CAD build for the part. Positions are in the model's coordinates, mm. Give positions to 0.01 mm unless a question says otherwise; leave off trailing zeros. Order: outer loops, then holes, each group sorted by start corner. A loop starts at its lowest first (then second) coordinate and runs counter-clockwise, first axis right, second up.
from build123d import *

# Parameters (mm, degrees)
BOSS_EXTRUDE1_DEPTH = 6.6


with BuildPart() as part:
    # Model → Boss-Extrude1 (new body)
    with BuildSketch(Plane.XY):
        with BuildLine():
            Line((-2.7, 21.1), (0, 21.1))
            Line((0, 21.1), (0, 0))
            Line((0, 0), (-76.35, 26.1117))
            Line((-76.35, 26.1117), (-100, 49.2))
            Line((-100, 49.2), (-100, 380.9))
            Line((-100, 380.9), (-97.5, 383.4))
            Line((-97.5, 383.4), (-80, 383.4))
            Line((-80, 383.4), (-61.92031318, 366.450293606))
            Line((-61.92031318, 366.450293606), (-69.443665597, 358.42538436))
            Line((-69.443665597, 358.42538436), (-70.599982066, 359.50943105))
            ThreePointArc((-70.599982066, 359.50943105), (-70.958073277, 359.644402505), (-71.306721232, 359.486633012))
            Line((-71.306721232, 359.486633012), (-74.042485748, 356.568484196))
            ThreePointArc((-74.042485748, 356.568484196), (-74.177457203, 356.210392984), (-74.01968771, 355.861745029))
            Line((-74.01968771, 355.861745029), (-72.863371242, 354.77769834))
            Line((-72.863371242, 354.77769834), (-75.941106322, 351.494780921))
            ThreePointArc((-75.941106322, 351.494780921), (-76.076077777, 351.13668971), (-75.918308284, 350.788041755))
            Line((-75.918308284, 350.788041755), (-74.057988413, 349.043991876))
            ThreePointArc((-74.057988413, 349.043991876), (-73.699897202, 348.909020421), (-73.351249247, 349.066789913))
            Line((-73.351249247, 349.066789913), (-70.273514167, 352.349707332))
            Line((-70.273514167, 352.349707332), (-69.117197698, 351.265660643))
            ThreePointArc((-69.117197698, 351.265660643), (-68.759106487, 351.130689188), (-68.410458532, 351.288458681))
            Line((-68.410458532, 351.288458681), (-65.674694016, 354.206607497))
            ThreePointArc((-65.674694016, 354.206607497), (-65.539722561, 354.564698709), (-65.697492054, 354.913346664))
            Line((-65.697492054, 354.913346664), (-66.853808523, 355.997393353))
            Line((-66.853808523, 355.997393353), (-59.330456105, 364.022302598))
            Line((-59.330456105, 364.022302598), (-45.469249226, 351.02742115))
            Line((-45.469249226, 351.02742115), (-42.733484711, 353.945569966))
            ThreePointArc((-42.733484711, 353.945569966), (-40.990244935, 354.73441743), (-39.199788878, 354.059560154))
            Line((-39.199788878, 354.059560154), (-31.904416837, 347.220148866))
            ThreePointArc((-31.904416837, 347.220148866), (-31.115569373, 345.47690909), (-31.790426649, 343.686453033))
            Line((-31.790426649, 343.686453033), (-34.526191164, 340.768304216))
            Line((-34.526191164, 340.768304216), (-20.664984286, 327.773422768))
            Line((-20.664984286, 327.773422768), (-28.188336703, 319.748513522))
            Line((-28.188336703, 319.748513522), (-29.344653172, 320.832560211))
            ThreePointArc((-29.344653172, 320.832560211), (-29.702744383, 320.967531667), (-30.051392338, 320.809762174))
            Line((-30.051392338, 320.809762174), (-32.787156854, 317.891613357))
            ThreePointArc((-32.787156854, 317.891613357), (-32.922128309, 317.533522146), (-32.764358816, 317.184874191))
            Line((-32.764358816, 317.184874191), (-31.608042348, 316.100827502))
            Line((-31.608042348, 316.100827502), (-34.685777428, 312.817910083))
            ThreePointArc((-34.685777428, 312.817910083), (-34.820748883, 312.459818871), (-34.66297939, 312.111170916))
            Line((-34.66297939, 312.111170916), (-32.802659519, 310.367121038))
            ThreePointArc((-32.802659519, 310.367121038), (-32.444568308, 310.232149583), (-32.095920353, 310.389919075))
            Line((-32.095920353, 310.389919075), (-29.018185273, 313.672836494))
            Line((-29.018185273, 313.672836494), (-27.861868804, 312.588789805))
            ThreePointArc((-27.861868804, 312.588789805), (-27.503777593, 312.45381835), (-27.155129638, 312.611587842))
            Line((-27.155129638, 312.611587842), (-24.419365122, 315.529736659))
            ThreePointArc((-24.419365122, 315.529736659), (-24.284393667, 315.88782787), (-24.44216316, 316.236475825))
            Line((-24.44216316, 316.236475825), (-25.598479629, 317.320522515))
            Line((-25.598479629, 317.320522515), (-18.075127211, 325.34543176))
            Line((-18.075127211, 325.34543176), (0, 308.4))
            Line((0, 308.4), (0, 295.7))
            Line((0, 295.7), (-2.7, 295.7))
            Line((-2.7, 295.7), (-2.7, 280.7))
            Line((-2.7, 280.7), (0, 280.7))
            Line((0, 280.7), (0, 270.3))
            Line((0, 270.3), (-11, 270.3))
            Line((-11, 270.3), (-11, 271.885))
            ThreePointArc((-11, 271.885), (-11.146446609, 272.238553391), (-11.5, 272.385))
            Line((-11.5, 272.385), (-15.5, 272.385))
            ThreePointArc((-15.5, 272.385), (-15.853553391, 272.238553391), (-16, 271.885))
            Line((-16, 271.885), (-16, 270.3))
            Line((-16, 270.3), (-20.5, 270.3))
            ThreePointArc((-20.5, 270.3), (-20.853553391, 270.153553391), (-21, 269.8))
            Line((-21, 269.8), (-21, 267.25))
            ThreePointArc((-21, 267.25), (-20.853553391, 266.896446609), (-20.5, 266.75))
            Line((-20.5, 266.75), (-16, 266.75))
            Line((-16, 266.75), (-16, 265.165))
            ThreePointArc((-16, 265.165), (-15.853553391, 264.811446609), (-15.5, 264.665))
            Line((-15.5, 264.665), (-11.5, 264.665))
            ThreePointArc((-11.5, 264.665), (-11.146446609, 264.811446609), (-11, 265.165))
            Line((-11, 265.165), (-11, 266.75))
            Line((-11, 266.75), (0, 266.75))
            Line((0, 266.75), (0, 232.2))
            Line((0, 232.2), (4, 232.2))
            ThreePointArc((4, 232.2), (5.767766953, 231.467766953), (6.5, 229.7))
            Line((6.5, 229.7), (6.5, 219.7))
            ThreePointArc((6.5, 219.7), (5.767766953, 217.932233047), (4, 217.2))
            Line((4, 217.2), (0, 217.2))
            Line((0, 217.2), (0, 209.166666667))
            Line((0, 209.166666667), (-2.7, 209.166666667))
            Line((-2.7, 209.166666667), (-2.7, 194.166666667))
            Line((-2.7, 194.166666667), (0, 194.166666667))
            Line((0, 194.166666667), (0, 155.975))
            Line((0, 155.975), (-11, 155.975))
            Line((-11, 155.975), (-11, 157.56))
            ThreePointArc((-11, 157.56), (-11.146446609, 157.913553391), (-11.5, 158.06))
            Line((-11.5, 158.06), (-15.5, 158.06))
            ThreePointArc((-15.5, 158.06), (-15.853553391, 157.913553391), (-16, 157.56))
            Line((-16, 157.56), (-16, 155.975))
            Line((-16, 155.975), (-20.5, 155.975))
            ThreePointArc((-20.5, 155.975), (-20.853553391, 155.828553391), (-21, 155.475))
            Line((-21, 155.475), (-21, 152.925))
            ThreePointArc((-21, 152.925), (-20.853553391, 152.571446609), (-20.5, 152.425))
            Line((-20.5, 152.425), (-16, 152.425))
            Line((-16, 152.425), (-16, 150.84))
            ThreePointArc((-16, 150.84), (-15.853553391, 150.486446609), (-15.5, 150.34))
            Line((-15.5, 150.34), (-11.5, 150.34))
            ThreePointArc((-11.5, 150.34), (-11.146446609, 150.486446609), (-11, 150.84))
            Line((-11, 150.84), (-11, 152.425))
            Line((-11, 152.425), (0, 152.425))
            Line((0, 152.425), (0, 122.633333333))
            Line((0, 122.633333333), (-2.7, 122.633333333))
            Line((-2.7, 122.633333333), (-2.7, 107.633333333))
            Line((-2.7, 107.633333333), (0, 107.633333333))
            Line((0, 107.633333333), (0, 91.2))
            Line((0, 91.2), (4, 91.2))
            ThreePointArc((4, 91.2), (5.767766953, 90.467766953), (6.5, 88.7))
            Line((6.5, 88.7), (6.5, 78.7))
            ThreePointArc((6.5, 78.7), (5.767766953, 76.932233047), (4, 76.2))
            Line((4, 76.2), (0, 76.2))
            Line((0, 76.2), (0, 54.35))
            Line((0, 54.35), (-11, 54.35))
            Line((-11, 54.35), (-11, 55.935))
            ThreePointArc((-11, 55.935), (-11.146446609, 56.288553391), (-11.5, 56.435))
            Line((-11.5, 56.435), (-15.5, 56.435))
            ThreePointArc((-15.5, 56.435), (-15.853553391, 56.288553391), (-16, 55.935))
            Line((-16, 55.935), (-16, 54.35))
            Line((-16, 54.35), (-20.5, 54.35))
            ThreePointArc((-20.5, 54.35), (-20.853553391, 54.203553391), (-21, 53.85))
            Line((-21, 53.85), (-21, 51.3))
            ThreePointArc((-21, 51.3), (-20.853553391, 50.946446609), (-20.5, 50.8))
            Line((-20.5, 50.8), (-16, 50.8))
            Line((-16, 50.8), (-16, 49.215))
            ThreePointArc((-16, 49.215), (-15.853553391, 48.861446609), (-15.5, 48.715))
            Line((-15.5, 48.715), (-11.5, 48.715))
            ThreePointArc((-11.5, 48.715), (-11.146446609, 48.861446609), (-11, 49.215))
            Line((-11, 49.215), (-11, 50.8))
            Line((-11, 50.8), (0, 50.8))
            Line((0, 50.8), (0, 36.1))
            Line((0, 36.1), (-2.7, 36.1))
            Line((-2.7, 36.1), (-2.7, 21.1))
        make_face()
        with BuildLine():
            Line((-89.8155254, 173.347348004), (-89.86349893, 172.952628674))
            Line((-89.86349893, 172.952628674), (-90.006760381, 172.584057561))
            ThreePointArc((-90.006760381, 172.584057561), (-92.000532075, 171.616009494), (-93.384262393, 173.347348004))
            Line((-93.384262393, 173.347348004), (-93.384262393, 189.222348004))
            ThreePointArc((-93.384262393, 189.222348004), (-92.000532075, 190.953686513), (-90.006760381, 189.985638446))
            Line((-90.006760381, 189.985638446), (-89.864204346, 189.619898255))
            Line((-89.864204346, 189.619898255), (-89.8155254, 189.222348004))
            Line((-89.8155254, 189.222348004), (-89.8155254, 173.347348004))
        make_face(mode=Mode.SUBTRACT)
    extrude(amount=BOSS_EXTRUDE1_DEPTH)


solid = part.part
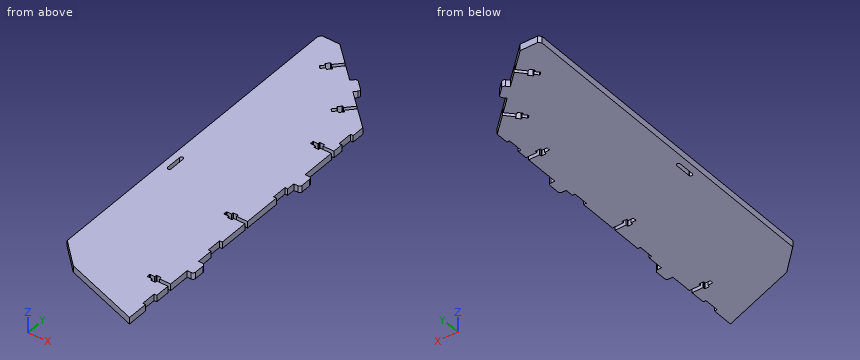
1. Saw through at A-A on y = 118.5. Give the cut face in (x, z).
2. Saw through at B-B on x = -51. Give the cut face in (y, z).
3. Pin check, flat tips, straight feed: P1, Ø3, axis at x = -14, z = 2, coming from the +Y side; P2, Ø1.2, axis at x = -12.5, z = 4.5, coming from the +Y side; P3, Ø0.8, axis at y = 156.5, z = 2, coming from the +X side. Stop position of each tip, or through.
4. Wall check: line 1 (Y direction, x = -13.5, z = 4.5) (3 decimals); line 2 (X direction, y = 173, z = 0.5); line 3 (Y direction, x = -19.5, z = 3.5) (3 decimals). Give the ranges that are in metal, low to high.
Reported:
1. outline: (-100, 0) - (-2.7, 0) - (-2.7, 6.6) - (-100, 6.6) - close
2. outline: (17.44, 0) - (356.21, 0) - (356.21, 6.6) - (17.44, 6.6) - close
3. P1: stops at y = 322.93
3. P2: stops at y = 320.68
3. P3: stops at x = 0
4. line 1: y = 4.617 to 48.715, 56.435 to 150.34, 158.06 to 264.665, 272.385 to 321.056
4. line 2: x = -100 to -93.35, -89.86 to 0
4. line 3: y = 6.669 to 50.8, 54.35 to 152.425, 155.975 to 266.75, 270.3 to 323.826
